CAD build for the part. Positions are in the model's coordinates, mm. Face numbers are marked on the shaded views. A direction names the side the tool comes from. Round coordinates to 2 decimals unless told otherwise and drop trailing zeros. Write each loop counter-clockwise with the first axis right and the second up, starting at its lowest first coordinate (ties: lowest second). Pieces come first, ordered by that corner, then holes. Notation, with made-up numbers: (79, 37.25) - (94, 37.25) arc R22 ccw to (94, 45.25) - close; hole circle Ø10 at (51, -32). An arc over 180 degrees is marked (long way). Put each result on its own line as item: value. Start each with the question number.
Item 1: Cut at A-A (z = -7.5). Give the cut face in (x, y).
Item 2: Drill centre lines: line 1 (X direction, y = -2.3, z = -7.5); line 2 (Z direction, x = 9.5, y = -1.25); line 3 (Y direction, x = 13.25, z = -22). Where is each one in solid material? Low to high. Write a range as from..to.
Item 3: Pin check, flat tips, straight feed: pin 1 Ø6 at (x, z) = (11, -10.5) entering from +Y; pin 2 Ø1.4 at (y, z) = (0.5, -15.5) entering from +X; pin 3 Ø3.5 at (x, y) = (12, -0.5) entering from -Z; pin 4 Ø10 at (y, z) = (6, -6.5) entering from +X. Stop position of each tip, or through.
Item 4: Cut at B-B (y = 3.5). Give the cut face in (x, z), and give its area (3 significant figures).
Item 5: Mould opens along X. For the marked faces 1, 2, 3 and 4 say: released by +X, released by -X, zero draft, split by the parting line, or undercut.
Item 6: Cut at C-C (x = 9.25). Give the cut face in (y, z), and give its area (3 significant figures).
Item 7: Cut at D-D (x = 15.5). Give the cut face in (y, z).
Item 8: 3-axis set-ups, long thin cutter, end or side, ignore diameter. For the marked faces 5, 6, 7 and 8: which of +Z, -Z, +X, -X, +Y, -Y reach the whole face in a straight line?
```python
from build123d import *

# Parameters (mm, degrees)
EXTRUDE_1_DEPTH     = 5
SKETCH_2_W          = 28
SKETCH_2_H          = 23
EXTRUDE_2_DEPTH     = 3
SKETCH_3_R          = 1.5
CUT_EXTRUDE_1_DEPTH = 44.809958913
SKETCH_4_R          = 3.5
SKETCH_4_R_2        = 1.25
CUT_EXTRUDE_2_DEPTH = 43.400619099
FILLET_3_R          = 14
FILLET_4_R          = 2
SKETCH_6_W          = 6
SKETCH_6_H          = 26.5
EXTRUDE_3_DEPTH     = 1.3
FILLET_5_R          = 2
FILLET_6_R          = 2
SKETCH_7_R          = 1.25
EXTRUDE_4_DEPTH     = 6
SKETCH_8_W          = 11
SKETCH_8_H          = 3.2
EXTRUDE_5_DEPTH     = 3
SKETCH_10_R         = 2.05
CUT_EXTRUDE_3_DEPTH = 3
CUT_EXTRUDE_4_DEPTH = 3
FILLET_7_R          = 1
FILLET_8_R          = 2
FILLET_9_R          = 2
CUT_EXTRUDE_5_DEPTH = 10
FILLET_10_R         = 4


with BuildPart() as part:
    # 草图1 → 凸台-拉伸1 (new body)
    with BuildSketch(Plane(origin=(0, 0, 0), x_dir=(1, 0, 0), z_dir=(0, 1, 0))):
        Polygon((0, 0), (8.25, 0), (18.75, 5.5), (18.75, 26.5), (0, 26.5), align=None)
    extrude(amount=-EXTRUDE_1_DEPTH)

    # 草图2 → 凸台-拉伸2 (add)
    with BuildSketch(Plane(origin=(18.75, 0, 0), x_dir=(0, 0, -1), z_dir=(1, 0, 0))):
        with Locations((19.5, 6.5)):
            Rectangle(SKETCH_2_W, SKETCH_2_H)
    extrude(amount=EXTRUDE_2_DEPTH)

    # 草图3 → 切除-拉伸1 (cut, through all)
    with BuildSketch(Plane(origin=(0, 0, 0), x_dir=(1, 0, 0), z_dir=(0, 1, 0))):
        with Locations(Location((9.25, 22.5, 0), (0, 0, 270))):
            Circle(SKETCH_3_R)
        with Locations(Location((9.25, 7.5, 0), (0, 0, 270))):
            Circle(SKETCH_3_R)
    extrude(amount=-CUT_EXTRUDE_1_DEPTH, mode=Mode.SUBTRACT)

    # 草图4 → 切除-拉伸2 (cut, through all)
    with BuildSketch(Plane.ZY.offset(-18.75)):
        with Locations((-17, 2)):
            Circle(SKETCH_4_R)
        with Locations((-9.9, 6.2)):
            Circle(SKETCH_4_R_2)
    extrude(amount=-CUT_EXTRUDE_2_DEPTH, mode=Mode.SUBTRACT)

    # 圆角3
    fillet_3_edges = [part.edges().sort_by_distance(p)[0] for p in [
        (20.25, 18, -5.5),
    ]]
    fillet(fillet_3_edges, radius=FILLET_3_R)

    # 圆角4
    fillet_4_edges = [part.edges().sort_by_distance(p)[0] for p in [
        (9.375, -5, -26.5),
    ]]
    fillet(fillet_4_edges, radius=FILLET_4_R)

    # 草图6 → 凸台-拉伸3 (add)
    with BuildSketch(Plane(origin=(0, 0, 0), x_dir=(1, 0, 0), z_dir=(0, 1, 0))):
        with Locations((3, 13.25)):
            Rectangle(SKETCH_6_W, SKETCH_6_H)
    extrude(amount=EXTRUDE_3_DEPTH)

    # 圆角5
    fillet_5_edges = [part.edges().sort_by_distance(p)[0] for p in [
        (0, -1.85, 0),
    ]]
    fillet(fillet_5_edges, radius=FILLET_5_R)

    # 圆角6
    fillet_6_edges = [part.edges().sort_by_distance(p)[0] for p in [
        (0, -0.85, -26.5),
        (0, -5, -13.25),
        (0, -4.414213562, -25.914213562),
        (5.125, -5, 0),
        (0.585786438, -5, -0.585786438),
    ]]
    fillet(fillet_6_edges, radius=FILLET_6_R)

    # 草图7 → 凸台-拉伸4 (add)
    with BuildSketch(Plane.ZY.offset(-18.75)):
        with Locations((-9.9, 6.2)):
            Circle(SKETCH_7_R)
    extrude(amount=-EXTRUDE_4_DEPTH)

    # 草图8 → 凸台-拉伸5 (add)
    with BuildSketch(Plane.ZY.offset(-18.75)):
        with Locations((-28, 19.6)):
            Rectangle(SKETCH_8_W, SKETCH_8_H)
    extrude(amount=-EXTRUDE_5_DEPTH)

    # 草图10 → 切除-拉伸3 (cut)
    with BuildSketch(Plane.ZY.offset(-18.75)):
        with Locations((-28.3, 11.203029343)):
            Circle(SKETCH_10_R)
    extrude(amount=-CUT_EXTRUDE_3_DEPTH, mode=Mode.SUBTRACT)

    # 草图11 → 切除-拉伸4 (cut)
    with BuildSketch(Plane.ZY.offset(-18.75)):
        with BuildLine():
            Line((-32.977113162, 9.140846799), (-29.820411226, -2.082982308))
            ThreePointArc((-29.820411226, -2.082982308), (-28.385182257, -4.188410986), (-25.969807465, -5))
            Line((-25.969807465, -5), (-33.5, -5))
            Line((-33.5, -5), (-33.5, 12.931284876))
            ThreePointArc((-33.5, 12.931284876), (-33.368662233, 11.018117903), (-32.977113162, 9.140846799))
        make_face()
    extrude(amount=-CUT_EXTRUDE_4_DEPTH, mode=Mode.SUBTRACT)

    # 圆角7
    fillet_7_edges = [part.edges().sort_by_distance(p)[0] for p in [
        (20.25, 18, -22.5),
    ]]
    fillet(fillet_7_edges, radius=FILLET_7_R)

    # 圆角8
    fillet_8_edges = [part.edges().sort_by_distance(p)[0] for p in [
        (20.25, 21.2, -22.5),
    ]]
    fillet(fillet_8_edges, radius=FILLET_8_R)

    # 圆角9
    fillet_9_edges = [part.edges().sort_by_distance(p)[0] for p in [
        (20.25, 21.2, -33.5),
    ]]
    fillet(fillet_9_edges, radius=FILLET_9_R)

    # 草图12 → 切除-拉伸5 (cut)
    with BuildSketch(Plane.ZY.offset(-18.75)):
        Polygon((-21.5, 18), (-33.5, 18), (-36.951224722, 21.933704181), (-20.790244944, 21.933704181), align=None)
    extrude(amount=-CUT_EXTRUDE_5_DEPTH, mode=Mode.SUBTRACT)

    # 圆角10
    fillet_10_edges = [part.edges().sort_by_distance(p)[0] for p in [
        (20.25, 18, -33.5),
    ]]
    fillet(fillet_10_edges, radius=FILLET_10_R)


solid = part.part
```
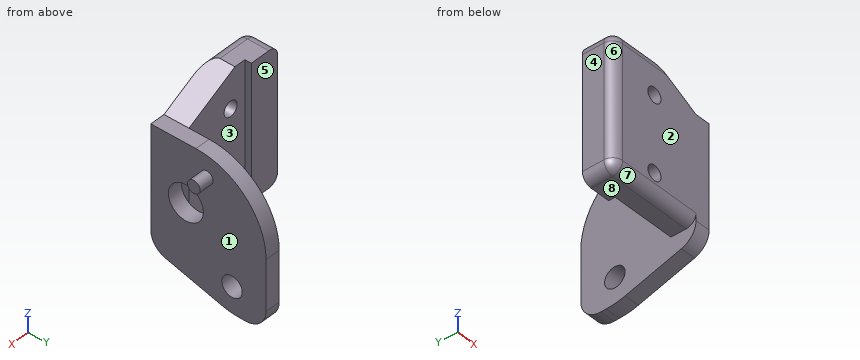
Output values:
1. outline: (0, -3) arc R2 ccw to (2, -5) - (7.75, -5) - (7.75, 0) - (6, 0) - (6, 1.3) - (0, 1.3) - close; (10.75, -5) - (21.75, -5) - (21.75, 11.21) - (18.75, 11.21) - (18.75, 0) - (10.75, 0) - close
2. line 1: 0..7.75, 10.75..21.75
2. line 2: -26.5..-23.98, -21.02..-8.98, -6.02..-0.65
2. line 3: -5..0
3. pin 1: y = 0
3. pin 2: x = 18.75
3. pin 3: z = -26.5
3. pin 4: x = 24.75
4. outline: (18.75, -31.39) - (21.75, -31.39) - (21.75, -20.16) - (18.75, -20.16) - close; (18.75, -13.84) - (21.75, -13.84) - (21.75, -5.5) - (18.75, -5.5) - close
4. area: 58.7 mm2
5. face 1: released by +X
5. face 2: zero draft
5. face 3: undercut
5. face 4: released by -X
6. outline: (-5, -24.5) arc R2 ccw to (-3, -26.5) - (0, -26.5) - (0, -24) - (-5, -24) - close; (-5, -21) - (0, -21) - (0, -9) - (-5, -9) - close; (-5, -6) - (0, -6) - (0, -0.52) - (-4.35, -0.52) arc R2 ccw to (-5, -2) - close
6. area: 98.7 mm2
7. outline: (-5, -24.5) arc R2 ccw to (-3, -26.5) - (0, -26.5) - (0, -3.8) - (-5, -3.8) - close
8. face 5: +Z, -Z, -X, +Y
8. face 6: +Z, -Z, -X, -Y
8. face 7: -Z, -X, -Y
8. face 8: -Z, -X, +Y, -Y
